Source: CAD feature listing. Evaluate the final solid. Frame: model axes, mm. Face numbers are marked on the shaded views. A direction names the side the tool comes from. Coordinates: 2 decimals unless noted, no trailing zeros. Order: outer loops, then holes, each group sorted by start corner. A loop starts at its lowest first (then second) coordinate and runs counter-clockwise, first axis right, second up.
```python
from build123d import *

# Parameters (mm, degrees)
SKETCH_1_R               = 125
SKETCH_1_R_2             = 20
SKETCH_1_W               = 30
SKETCH_1_H               = 30
EXTRUDE_1_DEPTH          = 10
SKETCH_1_3_W             = 30
SKETCH_1_3_H             = 30
EXTRUDE_2_DEPTH          = 25
SKETCH_7_R               = 5
EXTRUDE_3_DEPTH          = 2
EXTRUDE_START            = -2
SKETCH_4_R               = 5
EXTRUDE_4_DEPTH          = 2
PATTERN_CIRCULAR_1_COUNT = 4


with BuildPart() as part:
    # Sketch 1 → Extrude 1 (new body)
    with BuildSketch(Plane.XY):
        Circle(SKETCH_1_R)
        Circle(SKETCH_1_R_2, mode=Mode.SUBTRACT)
        with Locations((0, 95)):
            Rectangle(SKETCH_1_W, SKETCH_1_H, mode=Mode.SUBTRACT)
        with Locations((-95, 0)):
            Rectangle(SKETCH_1_W, SKETCH_1_H, mode=Mode.SUBTRACT)
        with Locations((0, -95)):
            Rectangle(SKETCH_1_W, SKETCH_1_H, mode=Mode.SUBTRACT)
        with Locations((95, 0)):
            Rectangle(SKETCH_1_W, SKETCH_1_H, mode=Mode.SUBTRACT)
    extrude(amount=EXTRUDE_1_DEPTH)

    # Sketch 1_3 → Extrude 2 (add)
    with BuildSketch(Plane.XY):
        with Locations((-95, 0)):
            Rectangle(SKETCH_1_3_W, SKETCH_1_3_H)
        with Locations((0, 95)):
            Rectangle(SKETCH_1_3_W, SKETCH_1_3_H)
        with Locations((95, 0)):
            Rectangle(SKETCH_1_3_W, SKETCH_1_3_H)
        with Locations((0, -95)):
            Rectangle(SKETCH_1_3_W, SKETCH_1_3_H)
    extrude(amount=EXTRUDE_2_DEPTH)

    # Sketch 7 → Extrude 3 (add)
    with BuildSketch(Plane(origin=(0, 15, 0), x_dir=(1, 0, 0), z_dir=(0, 1, 0))):
        with BuildLine():
            Line((80.290043894, -43.026337076), (80, -25))
            Line((80, -25), (110, -25))
            Line((110, -25), (107.550432268, -44.510860179))
            ThreePointArc((107.550432268, -44.510860179), (93.228538873, -56.470313397), (80.290043894, -43.026337076))
        make_face()
        with Locations(Location((93.972648447, -42.80618387, 0), (0, 0, 180))):
            Circle(SKETCH_7_R, mode=Mode.SUBTRACT)
    extrude_3 = extrude(amount=-EXTRUDE_3_DEPTH)

    # Sketch 4 → Extrude 4 (add)
    with BuildSketch(Plane.XZ.offset(15).offset(EXTRUDE_START)):
        with BuildLine():
            ThreePointArc((80.290043894, 43.026337076), (93.228538873, 56.470313397), (107.550432268, 44.510860179))
            Line((107.550432268, 44.510860179), (110, 25))
            Line((110, 25), (80, 25))
            Line((80, 25), (80.290043894, 43.026337076))
        make_face()
        with Locations(Location((93.972648447, 42.80618387, 0), (0, 0, 180))):
            Circle(SKETCH_4_R, mode=Mode.SUBTRACT)
    extrude_4 = extrude(amount=EXTRUDE_4_DEPTH)

    # Pattern Circular 1: Extrude 3, Extrude 4 ×4 about axis
    pattern_circular_1_axis = Axis((0, 0, 0), (0, 0, 1))
    add([extrude_3.rotate(pattern_circular_1_axis, i * 360 / PATTERN_CIRCULAR_1_COUNT) for i in range(1, PATTERN_CIRCULAR_1_COUNT)])
    add([extrude_4.rotate(pattern_circular_1_axis, i * 360 / PATTERN_CIRCULAR_1_COUNT) for i in range(1, PATTERN_CIRCULAR_1_COUNT)])


solid = part.part
```
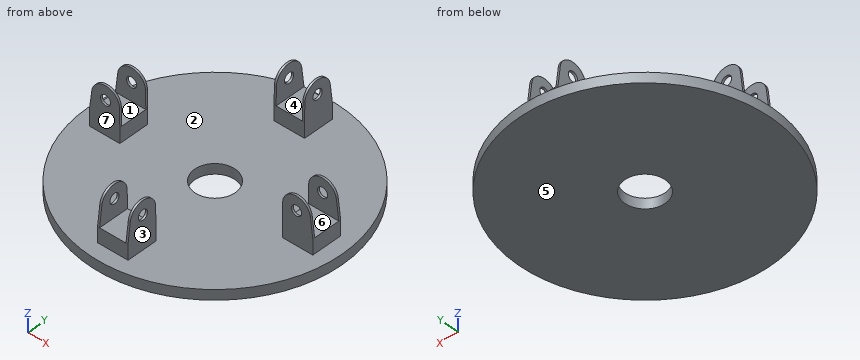
Q1. Section query A-A on x = 0. Output: boundary loops of the cut face in (y, z), plus the area to 3 significant figures.
Solutions:
outline: (-125, 0) - (-20, 0) - (-20, 10) - (-80, 10) - (-80, 25) - (-110, 25) - (-110, 10) - (-125, 10) - close; (20, 0) - (125, 0) - (125, 10) - (110, 10) - (110, 25) - (80, 25) - (80, 10) - (20, 10) - close
area: 3,000 mm2
Q2. Pin query (flat end, axial travel): P1, Ø24, axis at y = -89, z = 26, coming from the -X side; P2, Ø7.5, axis at x = 6, z = 17.5, coming from the -Y side; P3, Ø16.5, axis at y = 2.5, z = 15, coming from the -X side; P4, Ø6, axis at y = 93.97, z = 42.81, coming from the +X side (3 decimals). Return the tip coordinate at first contact, or that it passes through.
Solutions:
P1: stops at x = -15
P2: stops at y = -110
P3: stops at x = -125
P4: passes through
Q3. Section query D-D on x = 35. Output: boundary loops of the cut face in (y, z), plus the area to 3 significant figures.
Solutions:
outline: (-120, 0) - (120, 0) - (120, 10) - (-120, 10) - close
area: 2,400 mm2
Q4. Section query C-C on z = 14.5. Output: boundary loops of the cut face in (x, y).
Solutions:
outline: (-110, -15) - (-80, -15) - (-80, 15) - (-110, 15) - close; (-15, -110) - (15, -110) - (15, -80) - (-15, -80) - close; (-15, 80) - (15, 80) - (15, 110) - (-15, 110) - close; (80, -15) - (110, -15) - (110, 15) - (80, 15) - close
Q5. Pull-direction query (Y, two-part tool) for the marked faces 5, 6 and 7; classes: pulls with the +Y half, pulls with the -Y half, needs draft (parallel to the pull), parting line crosses it, or undercut.
Solutions:
face 5: needs draft
face 6: undercut
face 7: pulls with the -Y half
Q6. Set-up query: the marked faces 1, 2, 3 and 4. Return all of +Z, -Z, +X, -X, +Y, -Y with unobstructed straight access to the full face (end or side cutting, diameter ignored); none if empty.
Solutions:
face 1: +Z, +X, -X
face 2: +Z
face 3: +Z, +X, +Y, -Y
face 4: +Z, +Y, -Y
Q7. Material intervals for line 1 along Y through (x, z) = (108, 30); line 2 along Y through (x, z) = (6.5, 16); line 3 along Z through (x, y) = (-75.5, -54.5), sorted ascending.
Solutions:
line 1: y = -15 to -13, 13 to 15
line 2: y = -110 to -80, 80 to 110
line 3: z = 0 to 10
